```python
from build123d import *

# Parameters (mm, degrees)
SKETCH1_R           = 102.5
SKETCH1_R_2         = 94
SKETCH1_R_3         = 1.7
BOSS_EXTRUDE1_DEPTH = 3


with BuildPart() as part:
    # Sketch1 → Boss-Extrude1 (new body)
    with BuildSketch(Plane(origin=(0, 0, 0), x_dir=(1, 0, 0), z_dir=(0, 1, 0))):
        Circle(SKETCH1_R)
        Circle(SKETCH1_R_2, mode=Mode.SUBTRACT)
        with Locations((0, 97.974)):
            Circle(SKETCH1_R_3, mode=Mode.SUBTRACT)
        with Locations((48.987, 84.84797291)):
            Circle(SKETCH1_R_3, mode=Mode.SUBTRACT)
        with Locations((84.84797291, 48.987)):
            Circle(SKETCH1_R_3, mode=Mode.SUBTRACT)
        with Locations((97.974, 0)):
            Circle(SKETCH1_R_3, mode=Mode.SUBTRACT)
        with Locations((84.84797291, -48.987)):
            Circle(SKETCH1_R_3, mode=Mode.SUBTRACT)
        with Locations((48.987, -84.84797291)):
            Circle(SKETCH1_R_3, mode=Mode.SUBTRACT)
        with Locations((0, -97.974)):
            Circle(SKETCH1_R_3, mode=Mode.SUBTRACT)
        with Locations((-48.987, -84.84797291)):
            Circle(SKETCH1_R_3, mode=Mode.SUBTRACT)
        with Locations((-84.84797291, -48.987)):
            Circle(SKETCH1_R_3, mode=Mode.SUBTRACT)
        with Locations((-97.974, 0)):
            Circle(SKETCH1_R_3, mode=Mode.SUBTRACT)
        with Locations((-84.84797291, 48.987)):
            Circle(SKETCH1_R_3, mode=Mode.SUBTRACT)
        with Locations((-48.987, 84.84797291)):
            Circle(SKETCH1_R_3, mode=Mode.SUBTRACT)
    extrude(amount=BOSS_EXTRUDE1_DEPTH)


solid = part.part
```
Part model, mm, in its own coordinate system. Give positions to 0.01 mm unless a question says otherwise; leave off trailing zeros. Write each loop counter-clockwise with the first axis right and the second up, starting at its lowest first coordinate (ties: lowest second). Pieces come first, ordered by that corner, then holes. Notation, with made-up numbers: (2, -25.5) -> (24, -25.5) arc R25 ccw to (24, -4.5) -> close; hole circle Ø6 at (80.5, -37). An arc over 180 degrees is marked (long way). Put each result on its own line as item: value. Start each with the question number.
Item 1: Cut at B-B (x = 36). List the corners of the cut face in (y, z), then the cut area to 3 significant figures.
Item 2: Cut at A-A (z = 8). List the corners of the cut face in (x, y), then the cut area to 3 significant figures.
Item 3: Cut at C-C (y = 0.75). State how many separate pieces and enclosed holes the cut face has, then the cut area to 3 significant figures.
Item 4: Wall check: L1, parallel to Z at x = 0, y = 1.15; L2, parallel to Z at x = 2, y = 2.95. Give the ranges that are in metal, low to high. Write a range as [from, to].
Item 5: Pull direction Z, two halves, no side cores. Call faces 1 (the face through (89.659, 1.479, -28.235)), 2 (the face through (45, 0, 83)), 3 (the face through (-22.22, 1.479, 100.063)): pulls with the +Z half, pulls with the -Z half, needs draft (parallel to the pull), parting line crosses it, or undercut.
Item 6: Pin check, flat tip, straight feed: pin 1 Ø2 at (x, z) = (48.99, -84.85) entering from +Y. Stop position of the tip, or through.
Answer list:
1. outline: (0, -95.97) -> (3, -95.97) -> (3, -86.83) -> (0, -86.83) -> close; (0, 86.83) -> (3, 86.83) -> (3, 95.97) -> (0, 95.97) -> close
1. area: 54.8 mm2
2. outline: (-102.19, 0) -> (-93.66, 0) -> (-93.66, 3) -> (-102.19, 3) -> close; (93.66, 0) -> (102.19, 0) -> (102.19, 3) -> (93.66, 3) -> close
2. area: 51.2 mm2
3. separate pieces: 1
3. enclosed holes: 13
3. area: 5,140 mm2
4. L1: z = [-102.5, -99.67], [-96.27, -94], [94, 96.27], [99.67, 102.5]
4. L2: z = [-102.48, -93.98], [93.98, 102.48]
5. face 1: undercut
5. face 2: needs draft
5. face 3: parting line crosses it
6. pin 1: passes through
